```python
from build123d import *

# Parameters (mm, degrees)
SKETCH_1_R               = 2
EXTRUDE_1_DEPTH          = 50
CHAMFER_1_SIZE           = 15
EXTRUDE_2_DEPTH          = 50
CUT_EXTRUDE_1_DEPTH      = 50
CUT_EXTRUDE_1_DEPTH_BACK = 40
SKETCH_3_W               = 55
SKETCH_3_H               = 40
CUT_EXTRUDE_2_DEPTH      = 156.630973781
CUT_EXTRUDE_3_DEPTH      = 135.940727729
CHAMFER_2_SIZE           = 13.693


with BuildPart() as part:
    # 草图1 → 凸台-拉伸1 (new body)
    with BuildSketch(Plane(origin=(0, 0, 0), x_dir=(1, 0, 0), z_dir=(0, 1, 0))):
        Polygon((-35, 72), (-35, -42), (-15, -42), (20, -17), (20, 14.02557275), (20, 72), align=None)
        with Locations(Location((0, 0, 0), (0, 0, 270))):
            Circle(SKETCH_1_R, mode=Mode.SUBTRACT)
    extrude(amount=EXTRUDE_1_DEPTH)

    # 倒角1
    chamfer_1_edges = [part.edges().sort_by_distance(p)[0] for p in [
        (-35, 25, -72),
    ]]
    chamfer(chamfer_1_edges, length=CHAMFER_1_SIZE)

    # 草图2 → 凸台-拉伸2 (add)
    with BuildSketch(Plane(origin=(0, 50, 0), x_dir=(1, 0, 0), z_dir=(0, 1, 0))):
        with BuildLine():
            Line((-26, 39), (-26, -42))
            Line((-26, -42), (-35, -42))
            Line((-35, -42), (-35, 57))
            Line((-35, 57), (-20, 72))
            Line((-20, 72), (20, 72))
            Line((20, 72), (20, 65))
            Line((20, 65), (0, 65))
            ThreePointArc((0, 65), (-18.384776311, 57.384776311), (-26, 39))
        make_face()
    extrude(amount=EXTRUDE_2_DEPTH)

    # 草图3 → 切除-拉伸1 (cut, two sides: drawn at the far end of the back side and taken through both)
    with BuildSketch(Plane(origin=(0, 50, 0), x_dir=(1, 0, 0), z_dir=(0, 1, 0)).offset(-CUT_EXTRUDE_1_DEPTH_BACK)):
        with Locations((-7.5, 0)):
            Rectangle(SKETCH_3_W, SKETCH_3_H)
    extrude(amount=CUT_EXTRUDE_1_DEPTH + CUT_EXTRUDE_1_DEPTH_BACK, mode=Mode.SUBTRACT)

    # 草图4 → 切除-拉伸2 (cut, through all)
    with BuildSketch(Plane(origin=(0, 0, -72), x_dir=(-1, 0, 0), z_dir=(0, 0, -1))):
        Polygon((15, 0), (35, 40), (35, 0), align=None)
    extrude(amount=-CUT_EXTRUDE_2_DEPTH, mode=Mode.SUBTRACT)

    # 草图5 → 切除-拉伸3 (cut, through all)
    with BuildSketch(Plane(origin=(20, 0, 0), x_dir=(0, 0, -1), z_dir=(1, 0, 0))):
        Polygon((52, 0), (72, 0), (72, 40), align=None)
    extrude(amount=-CUT_EXTRUDE_3_DEPTH, mode=Mode.SUBTRACT)

    # 倒角2
    chamfer_2_edges = [part.edges().sort_by_distance(p)[0] for p in [
        (-21.25, 12.5, -58.25),
    ]]
    chamfer(chamfer_2_edges, length=CHAMFER_2_SIZE)


solid = part.part
```
Can you work these out from the model? Positions are in its coordinate system, mm. A direction names the side the tool comes from. Coordinates: 2 decimals unless noted, no trailing zeros. Loops run counter-clockwise (first coordinate to the right, second up) from the corner with the lowest first, then second, coordinate; pieces in that order, holes last.
1) For pin 1 (6 mm diameter, centred on x = 2, y = 21, fed in from +Z); pin 2 (10 mm diameter, centred on y = 25.5, z = -28.5, fed in from -X); pin 3 (17.5 mm diameter, centred on x = -5.5, z = 30.5, fed in from +Y), each with a flat end and sliding along its axis, tell me the tip position at first contact or that it passes through.
2) Which directions (+Z, -Z, +X, -X, +Y, -Y) give clear straight access to the entire face, cutting with the end or side of a thin tool? Please do faces 1 (the flat face through (-30, 100, 31)), 2 (the flat face through (-3, 50, -43)), 3 (the flat face through (0, 10, -5)).
3) Imagine slicing it at D-D on y = 87. List the corners of the cut face in (x, z) for me.
4) Imagine slicing it at C-C on z = -35.5. List the corners of the cut face in (x, y) for me, plus the area to 3 significant figures.
5) I need wall thicknesses on probe 1 along Y at (x, z) = (0, -29); probe 2 along Y at (x, z) = (-7, 8.5); probe 3 along Z at (x, y) = (8, 76.5). Which ranges of each line are inside material? Lowest first, please.
6) Imagine slicing it at B-B on z = 0. List the corners of the cut face in (x, y) for me, plus the area to 3 significant figures.
7) Imagine slicing it at A-A on y = 43. List the corners of the cut face in (x, z) for me, plus the area to 3 significant figures.
8) Thinking about a two-plate mould opening in Z: for faces 4 (the flat face through (-17.255, 19.72, -54.465)), 5 (the cylindrical face through (-2, 5, 0)), 6 (the flat face through (-26, 75, 31)), 7 (the flat face through (2.26, 24.65, 29.67)), which applies, pulls with the +Z half, pulls with the -Z half, needs draft (parallel to the pull), parting line crosses it, or undercut?
Completed:
1. pin 1: stops at z = 32
1. pin 2: stops at x = -30.25
1. pin 3: stops at y = 50
2. face 1: +Z, -Z, +X, -X, +Y
2. face 2: +Z, +X, +Y
2. face 3: +X, -X, +Y
3. outline: (-35, -57) - (-20, -72) - (20, -72) - (20, -65) - (0, -65) arc R26 cw to (-26, -39) - (-26, -20) - (-35, -20) - close; (-35, 20) - (-26, 20) - (-26, 42) - (-35, 42) - close
4. outline: (-35, 40) - (-15, 0) - (20, 0) - (20, 50) - (-26, 50) - (-26, 100) - (-35, 100) - close
4. area: 2,800 mm2
5. probe 1: y = 0 to 50
5. probe 2: y = 0 to 10
5. probe 3: z = -72 to -65
6. outline: (-20, 10) - (-15, 0) - (-2, 0) - (-2, 10) - close; (2, 0) - (20, 0) - (20, 10) - (2, 10) - close
6. area: 335 mm2
7. outline: (-35, -57) - (-20, -72) - (20, -72) - (20, -20) - (-35, -20) - close; (-35, 20) - (15.8, 20) - (-15, 42) - (-35, 42) - close
7. area: 3,530 mm2
8. face 4: pulls with the -Z half
8. face 5: undercut
8. face 6: needs draft
8. face 7: pulls with the +Z half
